from build123d import *
from OCP.BRepFilletAPI import BRepFilletAPI_MakeChamfer

# Parameters (mm, degrees)
SKETCH1_W               = 37.084
SKETCH1_H               = 24.638
BOSS_EXTRUDE1_DEPTH     = 6.858
CHAMFER2_SIZE           = 4.572
CHAMFER3_SIZE           = 2.54
CHAMFER3_SIZE2          = 4.399409051
CHAMFER4_SIZE           = 2.54
CHAMFER4_SIZE2          = 4.399409051
CUT_EXTRUDE1_DEPTH      = 46.04759998
CUT_EXTRUDE1_DEPTH_BACK = 2.54
SKETCH3_R               = 1


with BuildPart() as part:
    # Sketch1 → Boss-Extrude1 (new body)
    with BuildSketch(Plane.YZ):
        with Locations((18.542, -12.319)):
            Rectangle(SKETCH1_W, SKETCH1_H)
    extrude(amount=BOSS_EXTRUDE1_DEPTH)

    # Chamfer2
    chamfer2_edges = [part.edges().sort_by_distance(p)[0] for p in [
        (3.429, 0, 0),
        (3.429, 37.084, 0),
        (3.429, 37.084, -24.638),
        (3.429, 0, -24.638),
    ]]
    chamfer(chamfer2_edges, length=CHAMFER2_SIZE)

    # Chamfer3: one chamfer whose edges measure the first distance from different faces: ONE call of the kernel's chamfer builder (chamfer() names one face for all edges)
    chamfer3_edges_1 = [part.edges().sort_by_distance(p)[0] for p in [
        (6.858, 18.542, 0),
    ]]
    chamfer3_side_1 = [part.faces().sort_by_distance(p)[0] for p in [
        (3.429, 18.542, 0),
    ]]
    chamfer3_edges_2 = [part.edges().sort_by_distance(p)[0] for p in [
        (6.858, 18.542, -24.638),
    ]]
    chamfer3_side_2 = [part.faces().sort_by_distance(p)[0] for p in [
        (3.429, 18.542, -24.638),
    ]]
    chamfer3 = BRepFilletAPI_MakeChamfer(part.part.solid().wrapped)
    for e in chamfer3_edges_1:
        chamfer3.Add(CHAMFER3_SIZE, CHAMFER3_SIZE2, e.wrapped, chamfer3_side_1[0].wrapped)  # the first distance lies on this face
    for e in chamfer3_edges_2:
        chamfer3.Add(CHAMFER3_SIZE, CHAMFER3_SIZE2, e.wrapped, chamfer3_side_2[0].wrapped)  # the first distance lies on this face
    add(Compound.cast(chamfer3.Shape()), mode=Mode.REPLACE)

    # Chamfer4: one chamfer whose edges measure the first distance from different faces: ONE call of the kernel's chamfer builder (chamfer() names one face for all edges)
    chamfer4_edges_1 = [part.edges().sort_by_distance(p)[0] for p in [
        (6.858, 0, -12.319),
    ]]
    chamfer4_side_1 = [part.faces().sort_by_distance(p)[0] for p in [
        (3.429, 0, -12.319),
    ]]
    chamfer4_edges_2 = [part.edges().sort_by_distance(p)[0] for p in [
        (6.858, 37.084, -12.319),
    ]]
    chamfer4_side_2 = [part.faces().sort_by_distance(p)[0] for p in [
        (3.429, 37.084, -12.319),
    ]]
    chamfer4 = BRepFilletAPI_MakeChamfer(part.part.solid().wrapped)
    for e in chamfer4_edges_1:
        chamfer4.Add(CHAMFER4_SIZE, CHAMFER4_SIZE2, e.wrapped, chamfer4_side_1[0].wrapped)  # the first distance lies on this face
    for e in chamfer4_edges_2:
        chamfer4.Add(CHAMFER4_SIZE, CHAMFER4_SIZE2, e.wrapped, chamfer4_side_2[0].wrapped)  # the first distance lies on this face
    add(Compound.cast(chamfer4.Shape()), mode=Mode.REPLACE)

    # Sketch3 → Cut-Extrude1 (cut, two sides: drawn at the far end of the back side and taken through both)
    with BuildSketch(Plane(origin=(0, 0, 0), x_dir=(0, -1, 0), z_dir=(-1, 0, 0)).offset(-CUT_EXTRUDE1_DEPTH_BACK)):
        with Locations(Location((-8.542, -2.319, 0), (0, 0, 270))):
            Circle(SKETCH3_R)
        with Locations(Location((-8.542, -22.319, 0), (0, 0, 270))):
            Circle(SKETCH3_R)
        with Locations(Location((-28.542, -22.319, 0), (0, 0, 270))):
            Circle(SKETCH3_R)
        with Locations(Location((-28.542, -2.319, 0), (0, 0, 270))):
            Circle(SKETCH3_R)
    extrude(amount=CUT_EXTRUDE1_DEPTH + CUT_EXTRUDE1_DEPTH_BACK, mode=Mode.SUBTRACT)


solid = part.part
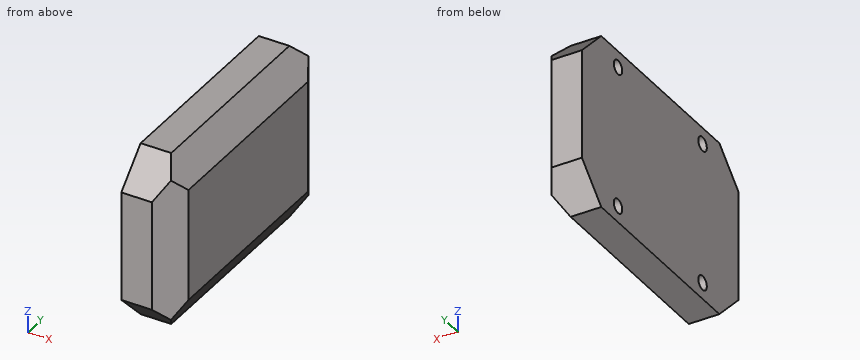
Part model, mm, in its own coordinate system. Give positions to 0.01 mm unless a question says otherwise; leave off trailing zeros. Loops run counter-clockwise (first coordinate to the right, second up) from the corner with the lowest first, then second, coordinate; pieces in that order, holes last. Notation, with made-up numbers: (56, 47) -> (81, 47) arc R8 ccw to (81, 61) -> close; hole circle Ø4 at (39.5, 35.5). An arc over 180 degrees is marked (long way). Write each question's results on one line, items separated by ' | '. Start each with the question number.
Q1. Band-saw the part on A-A on x = 1. List the corners of the cut face in (y, z).
Q2. Band-saw the part on B-B on y = 8. List the corners of the cut face in (x, z).
Q3. Pin check, flat tips, straight feed: P1, Ø2.5, axis at y = 28.542, z = -22.319, coming from the +X side; P2, Ø1.6, axis at y = 8.542, z = -22.319, coming from the +X side; P3, Ø1.5, axis at x = 6, z = -4, coming from the +Y side. Stop position of each tip, or through.
Q4. Band-saw the part on C-C on z = -13.5. List the corners of the cut face in (x, y), plus the area to 3 significant figures.
Q5. Band-saw the part on D-D on x = 5. List the corners of the cut face in (y, z).
Q6. Wall check: L1, parallel to Z at x = 1.5, y = 28; L2, parallel to Y at x = 4.5, z = -12; L3, parallel to Z at x = 6.25, y = 13. Give the ranges that are in metal, low to high.
Results are:
1) outline: (0, -20.07) -> (4.57, -24.64) -> (32.51, -24.64) -> (37.08, -20.07) -> (37.08, -4.57) -> (32.51, 0) -> (4.57, 0) -> (0, -4.57) -> close; hole circle Ø2 at (8.54, -22.32); hole circle Ø2 at (8.54, -2.32); hole circle Ø2 at (28.54, -22.32); hole circle Ø2 at (28.54, -2.32)
2) outline: (0, -24.64) -> (4.32, -24.64) -> (6.86, -20.24) -> (6.86, -4.4) -> (4.32, 0) -> (0, 0) -> (0, -1.48) -> (2.54, -1.48) -> (2.54, -3.16) -> (0, -3.16) -> (0, -21.48) -> (2.54, -21.48) -> (2.54, -23.16) -> (0, -23.16) -> close
3) P1: stops at x = 6.38 | P2: stops at x = 6.12 | P3: stops at y = 35.47
4) outline: (0, 0) -> (4.32, 0) -> (6.86, 4.4) -> (6.86, 32.68) -> (4.32, 37.08) -> (0, 37.08) -> close | area: 243 mm²
5) outline: (1.18, -21.25) -> (3.39, -23.46) -> (33.69, -23.46) -> (35.9, -21.25) -> (35.9, -3.39) -> (33.69, -1.18) -> (3.39, -1.18) -> (1.18, -3.39) -> close
6) L1: z = -24.64 to -23.16, -21.48 to -3.16, -1.48 to 0 | L2: y = 0.32 to 36.77 | L3: z = -21.29 to -3.35
